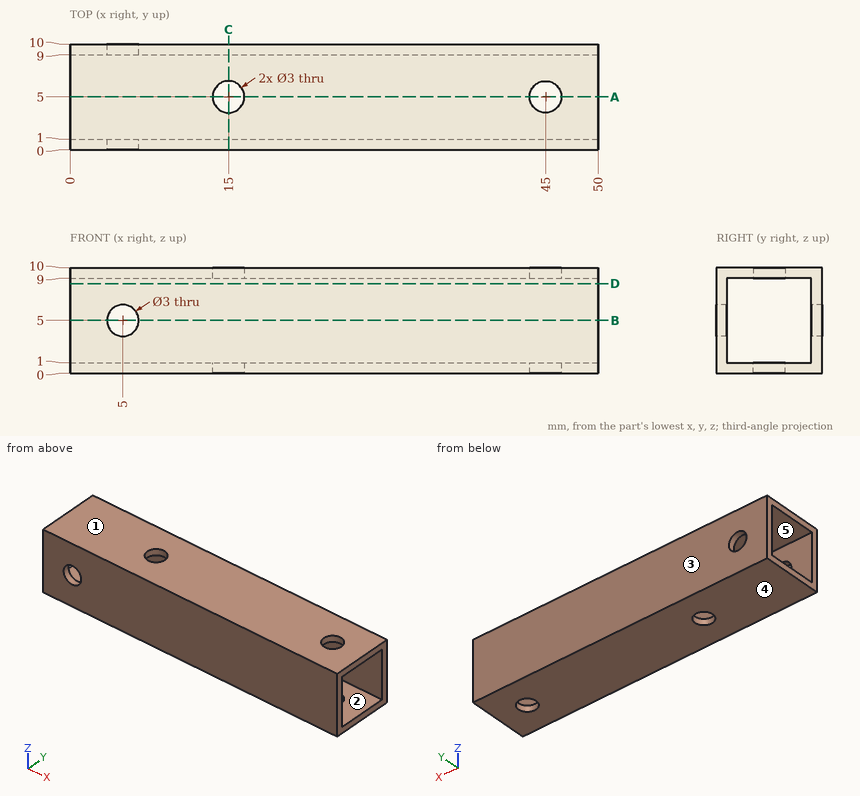
Drawing for the job (mm, zero at the part's lowest x, y, z). A direction names the side the tool comes from. Coordinates: 2 decimals unless noted, no trailing zeros. Order: outer loops, then holes, each group sorted by start corner. A loop starts at its lowest first (then second) coordinate and runs counter-clockwise, first axis right, second up.
Item 1: Band-saw the part on C-C on x = 15. List the corners of the cut face in (y, z).
Check sheet entries:
outline: (0, 0) - (3.5, 0) - (3.5, 1) - (1, 1) - (1, 9) - (3.5, 9) - (3.5, 10) - (0, 10) - close; (6.5, 0) - (10, 0) - (10, 10) - (6.5, 10) - (6.5, 9) - (9, 9) - (9, 1) - (6.5, 1) - close
Item 2: Drill centre lines: L1, parallel to Z at x = 22.5, y = 6.25; L2, parallel to Y at x = 15, z = 9.65. Where is each one in solid material? Low to high.
Check sheet entries:
L1: z = 0 to 1, 9 to 10
L2: y = 0 to 3.5, 6.5 to 10
Item 3: Band-saw the part on D-D on z = 8.5. List the corners of the cut face in (x, y).
Check sheet entries:
outline: (0, 0) - (50, 0) - (50, 1) - (0, 1) - close; (0, 9) - (50, 9) - (50, 10) - (0, 10) - close
Item 4: 3-axis set-ups, long thin cutter, end or side, ignore diameter. For the marked faces 1 and 2: which of +Z, -Z, +X, -X, +Y, -Y reach the whole face in a straight line?
Check sheet entries:
face 1: +Z, +X, -X, +Y, -Y
face 2: +X, -X
Item 5: Band-saw the part on A-A on y = 5. List the corners of the cut face in (x, z).
Check sheet entries:
outline: (0, 0) - (13.5, 0) - (13.5, 1) - (0, 1) - close; (0, 9) - (13.5, 9) - (13.5, 10) - (0, 10) - close; (16.5, 0) - (43.5, 0) - (43.5, 1) - (16.5, 1) - close; (16.5, 9) - (43.5, 9) - (43.5, 10) - (16.5, 10) - close; (46.5, 0) - (50, 0) - (50, 1) - (46.5, 1) - close; (46.5, 9) - (50, 9) - (50, 10) - (46.5, 10) - close
Item 6: Two-plate mould, pull along Y, no slides. Class the marked faces 3, 4 and 5: +Y half, -Y half, draft (parallel to the pull), parting line (faces both ways), or undercut.
Check sheet entries:
face 3: +Y half
face 4: draft
face 5: undercut
Item 7: Band-saw the part on B-B on z = 5. List the corners of the cut face in (x, y).
Check sheet entries:
outline: (0, 0) - (3.5, 0) - (3.5, 1) - (0, 1) - close; (0, 9) - (3.5, 9) - (3.5, 10) - (0, 10) - close; (6.5, 0) - (50, 0) - (50, 1) - (6.5, 1) - close; (6.5, 9) - (50, 9) - (50, 10) - (6.5, 10) - close
